from build123d import *

# Parameters (mm, degrees)
BOSS_EXTRUDE1_DEPTH = 403.86
CUT_EXTRUDE1_START  = -19.05
SKETCH3_R           = 22.86
CUT_EXTRUDE1_DEPTH  = 203.697116111
CUT_EXTRUDE2_START  = -19.05
SKETCH4_R           = 22.86
CUT_EXTRUDE2_DEPTH  = 203.697116111
CUT_EXTRUDE4_START  = -25.4
CUT_EXTRUDE4_DEPTH  = 353.06
SKETCH7_R           = 6.35
CUT_EXTRUDE5_DEPTH  = 76.2


with BuildPart() as part:
    # Sketch1 → Boss-Extrude1 (new body)
    with BuildSketch(Plane.XY):
        with BuildLine():
            Line((-10.998522628, 120.65), (-38.114105889, 167.615567884))
            Line((-38.114105889, 167.615567884), (-115.061446619, 123.19))
            Line((-115.061446619, 123.19), (-76.2, 55.88))
            Line((-76.2, 55.88), (-76.2, 0))
            Line((-76.2, 0), (76.2, 0))
            Line((76.2, 0), (76.2, 55.88))
            Line((76.2, 55.88), (115.061446619, 123.19))
            Line((115.061446619, 123.19), (38.114105889, 167.615567884))
            Line((38.114105889, 167.615567884), (10.998522628, 120.65))
            ThreePointArc((10.998522628, 120.65), (0, 114.3), (-10.998522628, 120.65))
        make_face()
    extrude(amount=-BOSS_EXTRUDE1_DEPTH)

    # Sketch3 → Cut-Extrude1 (cut, through all)
    with BuildSketch(Plane(origin=(82.108196401, 142.215567884, 0), x_dir=(0.866025404, -0.5, 0), z_dir=(0.5, 0.866025404, 0)).offset(CUT_EXTRUDE1_START)):
        with Locations((-6.374432116, 119.38)):
            Circle(SKETCH3_R)
        with Locations((-6.374432116, 231.14)):
            Circle(SKETCH3_R)
        with Locations((-6.374432116, 342.9)):
            Circle(SKETCH3_R)
    extrude(amount=-CUT_EXTRUDE1_DEPTH, mode=Mode.SUBTRACT)

    # Sketch4 → Cut-Extrude2 (cut, through all)
    with BuildSketch(Plane(origin=(-82.108196401, 142.215567884, 0), x_dir=(0.866025404, 0.5, 0), z_dir=(-0.5, 0.866025404, 0)).offset(CUT_EXTRUDE2_START)):
        with Locations((6.374432116, 63.5)):
            Circle(SKETCH4_R)
        with Locations((6.374432116, 175.26)):
            Circle(SKETCH4_R)
        with Locations((6.374432116, 287.02)):
            Circle(SKETCH4_R)
    extrude(amount=-CUT_EXTRUDE2_DEPTH, mode=Mode.SUBTRACT)

    # Sketch5 → Cut-Extrude4 (cut)
    with BuildSketch(Plane.XY.offset(CUT_EXTRUDE4_START)):
        with BuildLine():
            Line((-50.8, 0), (-50.8, 31.75))
            Line((-50.8, 31.75), (-26.311519178, 45.814017315))
            ThreePointArc((-26.311519178, 45.814017315), (0, 52.832), (26.311519178, 45.814017315))
            Line((26.311519178, 45.814017315), (50.8, 31.75))
            Line((50.8, 31.75), (50.8, 0))
            Line((50.8, 0), (-50.8, 0))
        make_face()
    extrude(amount=-CUT_EXTRUDE4_DEPTH, mode=Mode.SUBTRACT)

    # Sketch7 → Cut-Extrude5 (cut)
    with BuildSketch(Plane.XZ):
        with Locations((-63.5, -391.16)):
            Circle(SKETCH7_R)
        with Locations((63.5, -12.7)):
            Circle(SKETCH7_R)
    extrude(amount=-CUT_EXTRUDE5_DEPTH, mode=Mode.SUBTRACT)


solid = part.part
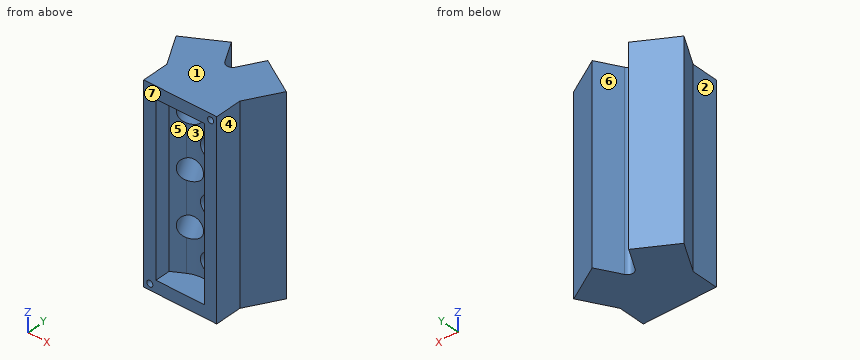
The listing builds one solid part. Answer for the finished solid, in the listing's coordinates (mm). Face numbers are marked on the shaded views. A direction names the side the tool comes from. Give positions to 0.01 mm unless a question says otherwise; leave off trailing zeros. Write each loop counter-clockwise with the first axis right and the second up, starting at its lowest first coordinate (ties: lowest second). Pieces come first, ordered by that corner, then holes.
Item 1: Which of the six approach directions +Z, -Z, +X, -X, +Y, -Y give full straight-line access (tool end or side, diameter ignored) to the marked faces 4, 5, 6 and 7?
Item 2: Section A-A, the plane y = 12.5 is taken. Write down the section's boundary in (x, z), plus the area to 3 significant figures.
Item 3: Determine the mould class of the marked faces 1, 2 and 3 for opening direction Z: released by +Z, released by -Z, zero draft, split by the parting line, or undercut.
Item 4: Flat-ended cylindrical pins translate along their axes: P1, Ø4, axis at y = 56, z = -80.5, coming from the -X side; P2, Ø3, axis at x = -29, z = -98, coming from the +Y side; P3, Ø3, axis at x = 24, z = -325, coming from the +Y side. Find the tip coordinate at first contact, or state that the pin passes through.
Item 5: Section D-D, the plane x = 65.5 is taken. Count the separate pieces of the cut face and the enclosed holes in it, plus the area to 3 significant figures.
Item 6: Section B-B, the plane z = -12.7 is taken. Write down the section's boundary in (x, y).
Item 7: Find the intervals of material crossed by line 1 along Z through (x, y) = (9, 25); line 2 along Z through (x, y) = (63, 18); line 3 along X through (y, z) = (27.5, -391.16), in increasing order.
Item 8: Section C-C, the plane y = 145 is taken. Write down the section's boundary in (x, z), plus the area to 3 significant figures.
Completed:
1. face 4: +Z, -Z, +X, -Y
1. face 5: -Y
1. face 6: +Z, -Z, +Y
1. face 7: +Z, -Z, +X, -X, -Y
2. outline: (-76.2, -403.86) - (76.2, -403.86) - (76.2, 0) - (-76.2, 0) - close; hole circle Ø12.7 at (-63.5, -391.16); hole (-50.8, -378.46) - (50.8, -378.46) - (50.8, -25.4) - (-50.8, -25.4) - close; hole circle Ø12.7 at (63.5, -12.7)
2. area: 25,400 mm2
3. face 1: released by +Z
3. face 2: zero draft
3. face 3: undercut
4. P1: stops at x = -77.42
4. P2: stops at y = 154.43
4. P3: stops at y = 145.77
5. separate pieces: 1
5. enclosed holes: 3
5. area: 55,000 mm2
6. outline: (-115.06, 123.19) - (-76.2, 55.88) - (-76.2, 0) - (57.15, 0) - (57.15, 76.2) - (69.85, 76.2) - (69.85, 0) - (76.2, 0) - (76.2, 55.88) - (115.06, 123.19) - (38.11, 167.62) - (11, 120.65) arc R12.7 cw to (-11, 120.65) - (-38.11, 167.62) - close
7. line 1: z = -403.86 to -378.46, -25.4 to 0
7. line 2: z = -403.86 to -19.03, -6.37 to 0
7. line 3: x = -76.2 to -69.85, -57.15 to 76.2
8. outline: (-77.29, -403.86) - (-25.06, -403.86) - (-25.06, 0) - (-77.29, 0) - close; (25.06, -403.86) - (77.29, -403.86) - (77.29, 0) - (25.06, 0) - close
8. area: 42,200 mm2
